Here's the drawing with two shaded views (mm, measured from the low corner). I have some questions. Round coordinates to 2 decimals unless told otherwise and drop trailing zeros. Order: outer loops, then holes, each group sorted by start corner. A loop starts at its lowest first (then second) coordinate and runs counter-clockwise, first axis right, second up. Notation, with made-up numbers: M 11,5 L 55,5 A19 cw 55,41 Z; hole C -6.5,74.25 d9. An arc over 180 degrees is marked long. One line per question, with ' | ' between items.
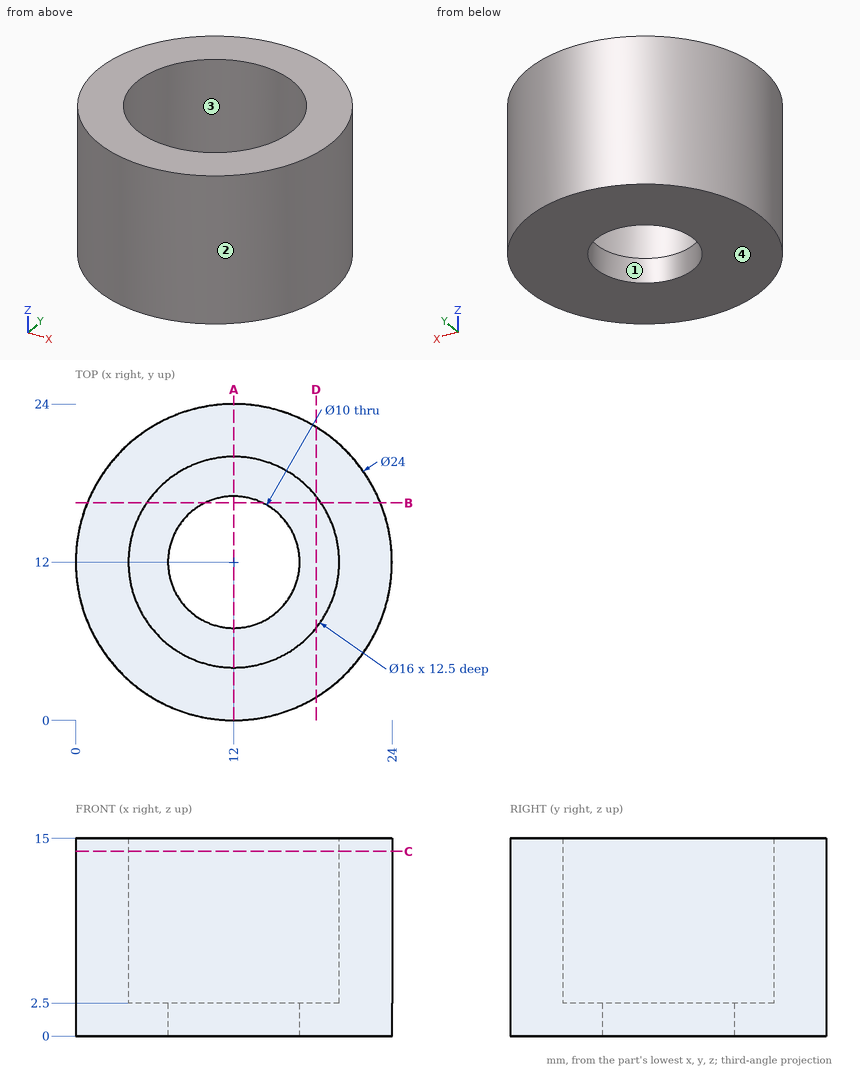
(1) If we section it at D-D on x = 18.25: Please give me the cut outline in (y, z), plus the area to 3 significant figures.
Final values:
outline: M 1.76,0 L 22.24,0 L 22.24,15 L 16.99,15 L 16.99,2.5 L 7.01,2.5 L 7.01,15 L 1.76,15 Z | area: 182 mm^2
(2) Thinking about a two-plate mould opening in X: for the marked faces 1, 2, 3 and 4, which applies, released by +X, released by -X, zero draft, split by the parting line, or undercut?
Final values:
face 1: undercut | face 2: split by the parting line | face 3: undercut | face 4: zero draft
(3) If we section it at B-B on y = 16.5: Please give me the cut outline in (x, z).
Final values:
outline: M 0.88,0 L 9.82,0 L 9.82,2.5 L 5.39,2.5 L 5.39,15 L 0.88,15 Z; M 14.18,0 L 23.12,0 L 23.12,15 L 18.61,15 L 18.61,2.5 L 14.18,2.5 Z
(4) If we section it at A-A on x = 12: Please give me the cut outline in (y, z).
Final values:
outline: M 0,0 L 7,0 L 7,2.5 L 4,2.5 L 4,15 L 0,15 Z; M 17,0 L 24,0 L 24,15 L 20,15 L 20,2.5 L 17,2.5 Z
(5) Please list where these lines run through material, in increasing order: probe 1 along X at (y, z) = (11.75, 13.25); probe 2 along X at (y, z) = (16.25, 6). Write a range as [from, to].
Final values:
probe 1: [0, 4], [20, 24] | probe 2: [0.78, 5.22], [18.78, 23.22]
(6) Will these pins go through, and if not, where does the flat tip stop? pin 1 Ø8 at (x, z) = (13.5, 12) entering from +Y; pin 2 Ø6 at (y, z) = (4, 3) entering from -X; pin 3 Ø6 at (y, z) = (5, 3.5) entering from +X; pin 4 Ø5 at (x, y) = (14, 14.5) entering from +Z.
Final values:
pin 1: y = 24 | pin 2: x = 1.09 | pin 3: x = 23.31 | pin 4: z = 2.5
(7) If we section it at C-C on z = 14: Please give me the cut outline in (x, y).
Final values:
outline: C 12,12 d24; hole C 12,12 d16
